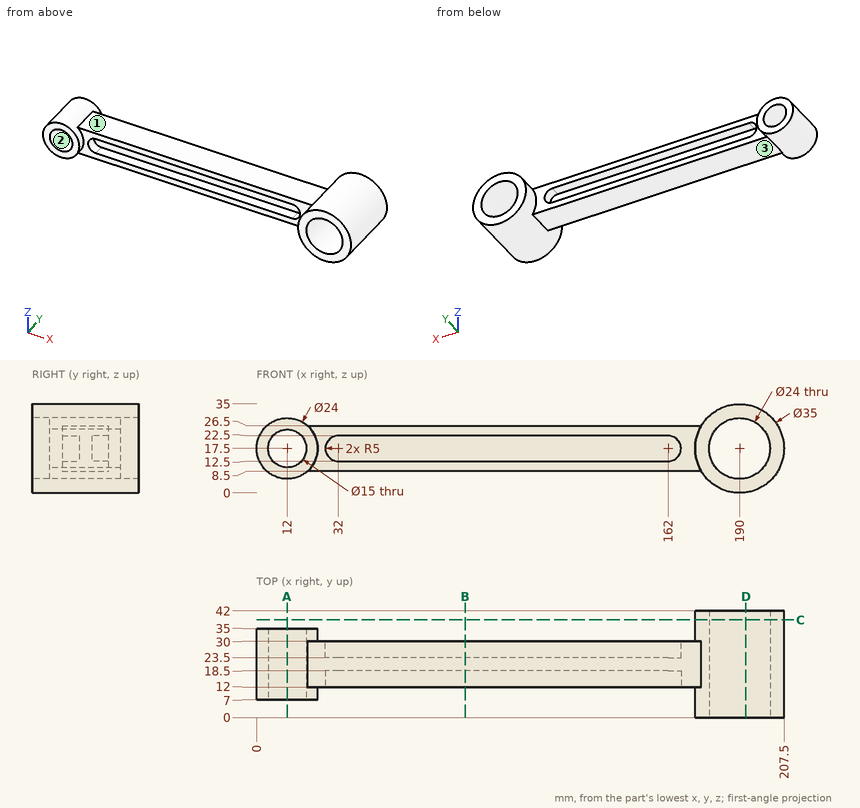
Can you work these out from the drawing? Everything is in mm from the part's minimum corner. A direction names the side the tool comes from. Give positions to 0.01 mm unless a question says otherwise; leave off trailing zeros. Order: outer loops, then holes, each group sorted by start corner. A loop starts at its lowest first (then second) coordinate and runs counter-clockwise, first axis right, second up. Notation, with made-up numbers: M 57,45 L 79,45 A18 cw 79,57 Z; hole C 80.25,-2 d6. An arc over 180 degrees is marked long. One line per question, with ' | ' between items.
1. I want a section at D-D (x = 192.5). List the corners of the cut face in (y, z) for me, and give its area (3 significant figures).
Results:
outline: M 0,0.18 L 42,0.18 L 42,5.76 L 0,5.76 Z; M 0,29.24 L 42,29.24 L 42,34.82 L 0,34.82 Z | area: 469 mm²
2. I want a section at C-C (y = 38.5). List the corners of the cut face in (x, z) for me.
Results:
outline: C 190,17.5 d35; hole C 190,17.5 d24
3. If I drill on line 1 (X direction, y = 13, z = 17); line 2 (X direction, y = 21.25, z = 17.5); line 3 (Z direction, x = 126.5, y = 15), over which ranges is the centre line in solid material (lowest first)?
Results:
line 1: 0.01 to 4.52, 19.48 to 27.03, 166.97 to 178.01, 201.99 to 207.49 | line 2: 0 to 4.5, 19.5 to 178, 202 to 207.5 | line 3: 8.5 to 12.5, 22.5 to 26.5
4. For the marked faces 1, 2 and 3, which set-ups out of +Z, -Z, +X, -X, +Y, -Y let a thin tool reach every point of the face, with its end or its side?
Results:
face 1: +Z, +Y, -Y | face 2: +Y, -Y | face 3: -Z, +Y, -Y
5. I want a section at B-B (x = 82). List the corners of the cut face in (y, z) for me, and give its area (3 significant figures).
Results:
outline: M 12,8.5 L 30,8.5 L 30,12.5 L 23.5,12.5 L 23.5,22.5 L 30,22.5 L 30,26.5 L 12,26.5 L 12,22.5 L 18.5,22.5 L 18.5,12.5 L 12,12.5 Z | area: 194 mm²
6. I want a section at A-A (x = 12). List the corners of the cut face in (y, z) for me, and give its area (3 significant figures).
Results:
outline: M 7,5.5 L 35,5.5 L 35,10 L 7,10 Z; M 7,25 L 35,25 L 35,29.5 L 7,29.5 Z | area: 252 mm²
7. I'm going to push flat-ended pins straight in: pin 1 (4 mm diameter, centred on y = 28, z = 29.5, fed in from -X); pin 2 (17 mm diameter, centred on x = 12, z = 17.5, fed in from -Y); pin 3 (4 mm diameter, centred on x = 40.5, z = 7, fed in from -Y). Where does each tip first touch, or does it pass through?
Results:
pin 1: x = 5.37 | pin 2: y = 7 | pin 3: y = 12
